Autodesk Inventor part; units mm, degrees
ref_plane "Work Plane1" through (0, 0, 0) normal (-0.7071, 0, -0.7071) x (0, 1, 0)
ref_plane "YZ Plane" through (0, 0, 0) normal (1, 0, 0) x (0, 1, 0)
ref_plane "XZ Plane" through (0, 0, 0) normal (0, 1, 0) x (-1, 0, 0)
sketch "Sketch1" plane through (0, 0, 0) normal (0, 1, 0) x (-1, 0, 0)
  line L0 (0, 0) -> (20, 0)
  line L1 (20, 0) -> (20, -50.8)
  line L2 (20, -50.8) -> (70.8, -50.8)
  line L3 (70.8, -50.8) -> (70.8, 0)
  line L4 (70.8, 0) -> (20, 0)
  line L5 (0, 0) -> (0, -70.808)
  line L6 (0, -70.808) -> (90.808, -70.808)
  line L7 (90.808, -70.808) -> (90.808, 20.008)
  line L8 (90.808, 20.008) -> (20, 20.008)
  line L9 (20, 20.008) -> (20, 0)
  dimension "d0" = 20
  dimension "d1" = 50.8
  dimension "d2" = 50.8
  dimension "d3" = 50.8
  dimension "d4" = 50.8
  dimension "d6" = 28.2899
  dimension "d7" = 28.2956
  dimension "d8" = 28.2956
  dimension "d11" = 20.008
extrude "Extrusion1" add sketch "Sketch1" along normal blind 155.0924
ref_plane "Work Plane1" through (0, 0, 0) normal (-0.7071, 0, -0.7071) x (0, 1, 0)
sketch "Sketch2" plane through (0, 0, 0) normal (-0.7071, 0, -0.7071) x (0, 1, 0)
  line L0 (155.0924, 21.7789) -> (155.0924, -14.1421)
  line L1 (155.0924, -14.1421) -> (52.705, -14.1421)
  line L2 (0, -14.1421) -> (155.0924, -14.1421)
  point P0 (0, 0)
  dimension "d15" = 102.3874
hole "Hole1" at (-10, 52.705, 10) direction (-0.7071, 0, -0.7071) diameter 12.7 depth 25.4
properties part number "LegHolderOutlet" material "Wood (Birch)"
Input: part model. Units: mm. Frame: model coordinates. A direction names the side the tool comes from. Coordinates: 2 decimals unless noted, no trailing zeros. Loops run counter-clockwise (first coordinate to the right, second up) from the corner with the lowest first, then second, coordinate; pieces in that order, holes last.
(1) First-contact query: pin 1 Ø12 at (x, z) = (-36.5, 10.5) entering from -Y; pin 2 Ø6 at (x, y) = (-5.5, 80.5) entering from +Z; pin 3 Ø5 at (y, z) = (95.5, 7.5) entering from +X. Flat tips, straight axial feed; report the tip coordinate or a pass-through.
(2) Section D-D on x = -8.5. Return the cut outline in (y, z), then the cut area to 3 significant figures.
(3) Set-up query: faces 5 (the face through (-46, 76, 0)), 6 (the face through (-24.55, 52.57, 4.43)), 7 (the face through (-56, 76, 20.008)), 8 (the face through (-20, 76, 10)). Return all of +Z, -Z, +X, -X, +Y, -Y with unobstructed straight access to the full face (end or side cutting, diameter ignored); none if empty.
(4) Section B-B on z = -16. Return the cut outline in (x, y).
(5) Material intervals for probe 1 along Z at (x, y) = (-46, 46.5); probe 2 along X at (y, z) = (15, -41); probe 3 along Z at (x, y) = (-16.5, 74.5), sorted ascending.
(6) Pull-direction query (X, two-part tool) for faces 1 (the face through (-90.808, 76, -26)), 2 (the face through (-45, 76, -50.8)), 3 (the face through (0, 76, -35)), 4 (the face through (-20, 76, -25)); classes: released by +X, released by -X, zero draft, split by the parting line, or undercut.
(7) Section A-A on x = -67.5. Return the cut outline in (y, z).
Data:
1. pin 1: stops at y = 0
1. pin 2: stops at z = 0
1. pin 3: stops at x = -20
2. outline: (0, -70.81) - (155.09, -70.81) - (155.09, 0) - (0, 0) - close
2. area: 11,000 mm2
3. face 5: +Y, -Y
3. face 6: +X
3. face 7: +Z, +X, -X, +Y, -Y
3. face 8: +Z, +X, +Y, -Y
4. outline: (-90.81, 0) - (-70.8, 0) - (-70.8, 155.09) - (-90.81, 155.09) - close; (-20, 0) - (0, 0) - (0, 155.09) - (-20, 155.09) - close
5. probe 1: z = -70.81 to -50.8, 0 to 20.01
5. probe 2: x = -90.81 to -70.8, -20 to 0
5. probe 3: z = -70.81 to 0
6. face 1: released by -X
6. face 2: undercut
6. face 3: released by +X
6. face 4: undercut
7. outline: (0, -70.81) - (155.09, -70.81) - (155.09, -50.8) - (0, -50.8) - close; (0, 0) - (155.09, 0) - (155.09, 20.01) - (0, 20.01) - close
